Input: dimensioned drawing with shaded views. Units: mm. Origin: part minimum x, y, z. Give positions to 0.01 mm unless a question says otherwise; leave off trailing zeros. Write each loop counter-clockwise with the first axis right and the second up, starting at its lowest first coordinate (ties: lowest second). Pieces come first, ordered by that corner, then holes. Notation, with made-up numbers: M 83,-37.5 L 136,-37.5 A16 cw 136,-22.5 Z; hole C 12.5,-17.75 d1. An arc over 180 degrees is marked long. Answer as a JSON object with one key per item and string values.
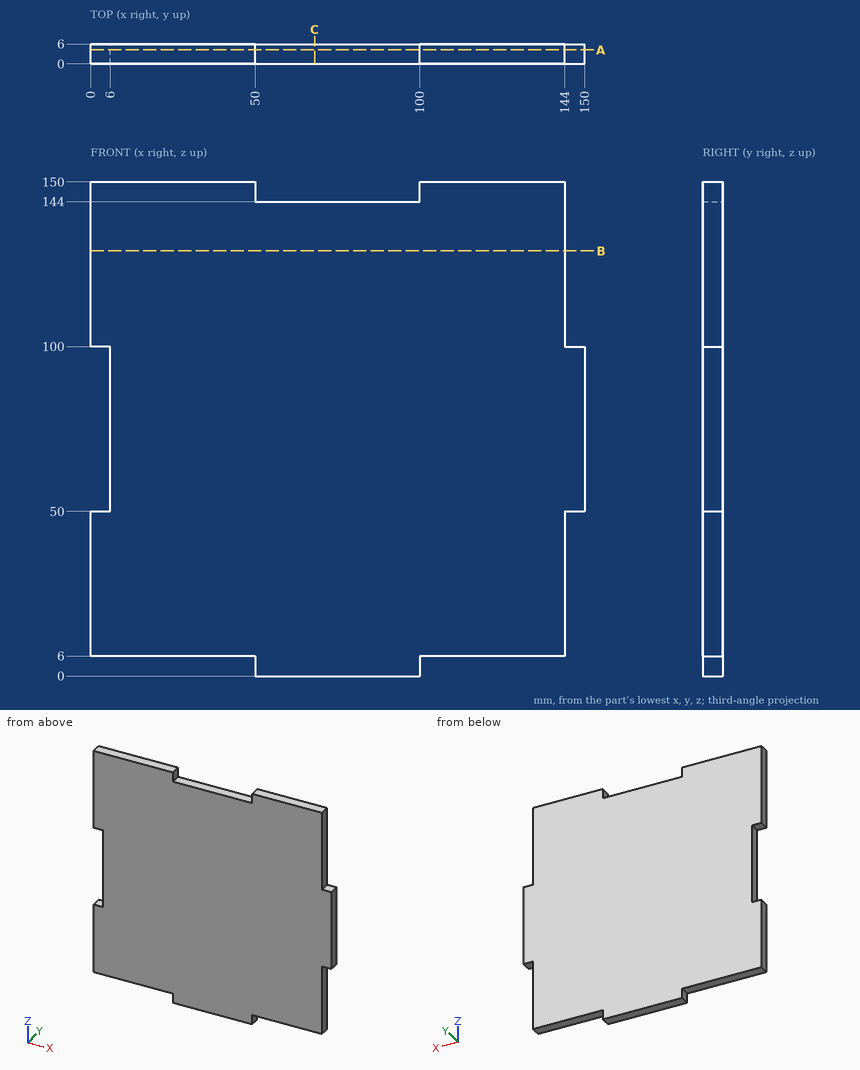
1) Line query: line 1 (Z direction, x = 8.5, y = 4.75); line 2 (Z direction, x = 87, y = 5.5). Output: solid intervals per line, ascending. Write a range as from..to.
Geometry check:
{"line 1": "z = 6..150", "line 2": "z = 0..144"}
2) Cut plane B-B on z = 129. Return loops of the section in (x, y).
Geometry check:
{"outline": "M 0,0 L 144,0 L 144,6 L 0,6 Z"}
3) Cut plane C-C on x = 68. Return loops of the section in (y, z).
Geometry check:
{"outline": "M 0,0 L 6,0 L 6,144 L 0,144 Z"}
4) Cut plane A-A on y = 4.2. Return loops of the section in (x, z).
Geometry check:
{"outline": "M 0,6 L 50,6 L 50,0 L 100,0 L 100,6 L 144,6 L 144,50 L 150,50 L 150,100 L 144,100 L 144,150 L 100,150 L 100,144 L 50,144 L 50,150 L 0,150 L 0,100 L 6,100 L 6,50 L 0,50 Z"}
5) Contact query for flat-ended pins moving along their axis: P1, Ø3, axis at x = 64.5, y = 3.5, coming from the +Z side; P2, Ø2, axis at x = 48.5, y = 1, coming from the -Z side; P3, Ø1.8, axis at y = 3, z = 3, coming from the -X side. Output: stop coordinate, or through.
Geometry check:
{"P1": "stops at z = 144", "P2": "stops at z = 6", "P3": "stops at x = 50"}
